Autodesk Inventor part; units mm, degrees
ref_plane "YZ Plane" through (0, 0, 0) normal (1, 0, 0) x (0, 1, 0)
ref_plane "XZ Plane" through (0, 0, 0) normal (0, 1, 0) x (-1, 0, 0)
ref_plane "XY Plane" through (0, 0, 0) normal (0, 0, 1) x (1, 0, 0)
sketch "Sketch1" plane through (0, 0, 0) normal (0, 0, 1) x (1, 0, 0)
  line L0 (-7, 8.5625) -> (0, 8.5625)
  line L1 (0, 8.5625) -> (0, -8.5625)
  line L2 (0, -8.5625) -> (-7, -8.5625)
  line L3 (-7, -8.5625) -> (-7, 8.5625)
  point P0 (0, 0)
  dimension "d0" = 0
  dimension "FRONT_LENGTH" = 7
  dimension "WIDTH" = 17.125
  dimension "d3" = 8.5625
extrude "Extrusion1" add sketch "Sketch1" along normal blind 28.95
sketch "Sketch2" plane through (0, 0, 0) normal (0, 0, 1) x (1, 0, 0)
  line L0 (0, -8.5625) -> (0, 8.5625)
  line L1 (0, 8.5625) -> (12, 8.5625)
  line L2 (12, 8.5625) -> (12, -8.5625)
  line L3 (12, -8.5625) -> (0, -8.5625)
  line L4 (0, -8.5625) -> (0, 8.5625)
  point P0 (0, 0)
  point P1 (0, -8.5625)
  dimension "d6" = 17.125
  dimension "BACK_LENGTH" = 12
sketch "Sketch3" plane through (-7, -8.5625, 0) normal (-1, 0, 0) x (0, 0, 1)
  circle A0 centre (19.05, 8.5625) radius 6.5625
  circle A1 centre (19.05, 8.5625) radius 7.0705
  circle A2 centre (13.8389, 10.4592) radius 1.525
  circle A3 centre (13.8389, 6.6658) radius 1.525
  line L0 (13.8389, 10.4592) -> (19.05, 8.5625)
  line L1 (19.05, 8.5625) -> (13.8389, 6.6658)
  line L2 (19.05, 8.5625) -> (0, 8.5625)
  point P0 (12.4059, 6.1442)
  point P1 (13.4136, 5.2013)
  point P2 (13.4136, 11.9237)
  point P3 (12.4059, 10.9808)
  dimension "d8" = 0
  dimension "MIRROR_HOLE" = 13.125
  dimension "d10" = 14.141
  dimension "d11" = 3.05
  dimension "d12" = 3.05
  dimension "d13" = 19.05
  dimension "d14" = 20
  dimension "d15" = 20
  dimension "d16" = 0
  dimension "d17" = 0
extrude "Extrusion2" cut sketch "Sketch3" against normal blind 6 contours A0 A3 L1 L0 A2 | A2 A0 | A0 A2 | A3 A0 | A0 A3 | A2 L0 L2 A0 | A0 L2 A1 A2 | A3 A1 L2 A0 | A0 L2 L1 A3
sketch "Sketch5" plane through (-1, -8.5625, 0) normal (-1, 0, 0) x (0, 0, 1)
  circle A0 centre (19.05, 8.5625) radius 6.0625
  point P0 (0, 8.5625)
  dimension "d20" = 0
  dimension "d21" = 19.05
  dimension "d22" = 12.125
extrude "Extrusion3" cut sketch "Sketch5" against normal up to surface (1 mm away)
extrude "Extrusion4" add sketch "Sketch2" along normal blind 5
sketch "Sketch6" plane through (0, 0, 5) normal (0, 0, 1) x (1, 0, 0)
  point P0 (0, 0)
  point P1 (6, 0)
  dimension "d27" = 0
  dimension "d28" = 6
hole "Hole1" at (6, 0, 5) direction (0, 0, -1) diameter 4.5 depth 5 counterbore diameter 8 counterbore depth 1.5
sketch "Sketch7" plane through (0, 0, 0) normal (0, 0, -1) x (-1, 0, 0)
  circle A0 centre (-6, 0) radius 2.25
  line L0 (-6, 5.498) -> (-6, 4.502) construction
  line L1 (-7.05, 5.498) -> (-7.05, 4.502)
  line L2 (-4.95, 4.502) -> (-4.95, 5.498)
  arc A1 (-4.95, 5.498) -> (-7.05, 5.498) centre (-6, 5.498) ccw
  arc A2 (-7.05, 4.502) -> (-4.95, 4.502) centre (-6, 4.502) ccw
  point P0 (0, 0)
  point P1 (-6, -5)
  point P2 (-6, 5)
  dimension "d36" = 0
  dimension "d37" = 0
  dimension "d38" = 5
  dimension "d39" = 5
  dimension "d63" = 1.05
  dimension "d64" = 0.996
hole "Hole2" at (6, -5, 0) direction (0, 0, 1) diameter 2.1 depth 2.1
sketch "Sketch8" plane through (0, 0, 28.95) normal (0, 0, 1) x (1, 0, 0)
  point P0 (0, 0)
  point P1 (-3.5, 0)
  dimension "d47" = 3.5
  dimension "d48" = 0
hole "Hole4" at (-3.5, 0, 28.95) direction (0, 0, -1) diameter 2.1565 end up to surface
extrude "Extrusion5" cut sketch "Sketch7" against normal blind 2.1 contours A1 L2 A2 L1
chamfer "Chamfer1" distance 1 angle 45 4 edges at (-3.5, -8.5625, 28.95) (-3.5, 8.5625, 28.95) (12, -8.5625, 2.5) (12, 8.5625, 2.5)
sketch "Sketch9" plane through (12, -7.5625, 0) normal (1, 0, 0) x (0, 0, -1)
  circle A0 centre (12.35, 7.5625) radius 12.7
  point P0 (0, 7.5625)
  dimension "d70" = 0
  dimension "d71" = 25.4
  dimension "d72" = 12.35
extrude "Extrusion6" cut sketch "Sketch9" against normal up to surface (19 mm away)
equation "\"WIDTH\" = MIRROR_HOLE + 2 * MIN_WALL_THICKNESS"
equation "\"d13\" = BEAM_HEIGHT"
equation "\"d6\" = WIDTH"
equation "\"BEAM_HEIGHT\" = 19.05"
equation "\"MIN_WALL_THICKNESS\" = 2"
equation "\"OPTICS_DIAMETER\" = 12.7"
equation "\"TOLERANCE\" = 0.05"
properties part number "ADAPTER_fixed-mirror-BH19.05-D12.7"
Model file for the job. Use its own axes, mm. A direction names the side the tool comes from. Round coordinates to 2 decimals unless told otherwise and drop trailing zeros. Loops run counter-clockwise (first coordinate to the right, second up) from the corner with the lowest first, then second, coordinate; pieces in that order, holes last. Notation, with made-up numbers: M 68,-3 L 88,-3 A16 ccw 88,25 Z; hole C 61.25,11 d11. An arc over 180 degrees is marked long. Put each result on its own line as item: value. Start each with the question number.
Item 1: Cut at C-C (x = 6). List the corners of the cut face in (y, z), then the cut area to 3 significant figures.
Item 2: Cut at A-A (z = 19.05). List the corners of the cut face in (x, y), then the cut area to 3 significant figures.
Item 3: Cut at B-B (y = 0). List the corners of the cut face in (x, z), then the cut area to 3 significant figures.
Item 4: 3-axis set-ups, long thin cutter, end or side, ignore diameter. For faces 1 (the face through (-4.042, -3.003, 12.79)), 2 (the face through (7.05, 5, 1)), 3 (the face through (9.905, 0.867, 4.24)): which of +Z, -Z, +X, -X, +Y, -Y reach the whole face in a straight line?
Item 5: Drop flat-ended pins along their axis: P1, Ø3, axis at x = -3.5, y = 0, coming from the -Z side; P2, Ø6, axis at x = 7.5, y = -0.5, coming from the +Z side. Give the stop position or say it passes through.
Item 6: Mould opens along Z. For faces 4 (the face through (6.023, 3.452, 1.035)), 5 (the face through (-3.45, -8.07, 28.44)), 6 (the face through (-1, -2, 13)) say: released by +Z, released by -Z, zero draft, split by the parting line, or undercut.
Item 7: Cut at D-D (y = -5.25). List the corners of the cut face in (x, z), then the cut area to 3 significant figures.
Item 8: Drill centre lines: line 1 along X through (y, z) = (-5, 0.9); line 2 along X through (y, z) = (0, 28.1); line 3 along Z through (x, y) = (4.5, -3). Where is each one in solid material? Low to high.
Answer block:
1. outline: M -8.56,0 L -6.05,0 L -6.05,2.1 L -3.95,2.1 L -3.95,0 L -2.96,0 A12.7 cw -2.25,0.15 L -2.25,3.5 L -4,3.5 L -4,5 L -8.56,5 Z; M 2.25,0.15 A12.7 cw 2.96,0 L 3.45,0 L 3.45,2.1 L 6.55,2.1 L 6.55,0 L 8.56,0 L 8.56,5 L 4,5 L 4,3.5 L 2.25,3.5 Z
1. area: 46.9 mm2
2. outline: M -7,-8.56 L 0,-8.56 L 0,-6.06 L -1,-6.06 L -1,-6.56 L -7,-6.56 Z; M -7,6.56 L -1,6.56 L -1,6.06 L 0,6.06 L 0,8.56 L -7,8.56 Z
2. area: 29.0 mm2
3. outline: M -7,0.35 L 3.75,0.35 L 3.75,3.5 L 2,3.5 L 2,5 L 0,5 L 0,12.99 L -1,12.99 L -1,11.98 L -7,11.98 Z; M -7,25.61 L -4.58,25.61 L -4.58,28.95 L -7,28.95 Z; M -2.42,25.61 L -1,25.61 L -1,25.11 L 0,25.11 L 0,28.95 L -2.42,28.95 Z; M 8.25,0.35 L 12,0.35 L 12,5 L 10,5 L 10,3.5 L 8.25,3.5 Z
3. area: 129 mm2
4. face 1: -X
4. face 2: -Z
4. face 3: +Z
5. P1: z = 0.26
5. P2: z = 5
6. face 4: zero draft
6. face 5: released by +Z
6. face 6: undercut
7. outline: M -7,0 L 4.98,0 L 4.98,2.1 L 7.02,2.1 L 7.02,0 L 12,0 L 12,5 L 0,5 L 0,16.02 L -1,16.02 L -1,15.11 L -7,15.11 Z; M -7,22.99 L -1,22.99 L -1,22.08 L 0,22.08 L 0,28.95 L -7,28.95 Z
7. area: 205 mm2
8. line 1: -7 to 4.95, 7.05 to 12
8. line 2: -7 to -4.58, -2.42 to 0
8. line 3: 0 to 3.5
